Model file for the job. Use its own axes, mm. A direction names the side the tool comes from. Round coordinates to 2 decimals unless told otherwise and drop trailing zeros. Loops run counter-clockwise (first coordinate to the right, second up) from the corner with the lowest first, then second, coordinate; pieces in that order, holes last. Notation, with made-up numbers: M -28,-2 L -17,-2 A21 cw -17,25 Z; hole C 22,58 d5. An arc over 180 degrees is marked long. Use a Markdown table: item, result. Add a question column.
Q1. Cut at A-A (y = 0). Give the cut face in (x, z).
Q2. Mould opens along Y. For faces 6 (the face through (12, 16, 5)), 7 (the face through (5, -7, 29.4)), 8 (the face through (-1, 15, 11.6)) say: +Y half, -Y half, draft (parallel to the pull), parting line (faces both ways), or undercut.
Q3. Pin check, flat tips, straight feed: pin 1 (0.9 mm diameter, centred on x = 6, y = -3, fed in from +Z); pin 2 (5 mm diameter, centred on x = -12.5, z = 8.5, fed in from +Y); pin 3 (8 mm diameter, centred on y = -1, z = 25.5, fed in from +X). Stop position of each tip, or through.
Q4. Probe line 1 (X direction, y = -10, z = 8.75); line 2 (Y direction, x = 0, z = 7); line 3 (Y direction, x = 2, z = 21.75). List the from-to ranges inside material, lowest first. Write a range as from..to.
Q5. Cut at B-B (z = 8.5). Give the cut face in (x, y) (3 decimals).
Q6. Tool access for faces 1 (the face through (-3.5, -6, 28)), 2 (the face through (-1.5, 16.164, 11.5)), 3 (the face through (1.5, 16.164, 11.5)), 4 (the face through (-4.75, 7, 28)), 5 (the face through (6, 0, 9)): list every direction of +Z, -Z, +X, -X, +Y, -Y with a clear straight run to the whole face (end or side of a thin tool).
from build123d import *

# Parameters (mm, degrees)
SKETCH1_R           = 20
SKETCH1_R_2         = 4.75
BOSS_EXTRUDE1_DEPTH = 11
SKETCH2_W           = 13.186598354
SKETCH2_H           = 1
SKETCH2_W_2         = 3
SKETCH2_H_2         = 26.426474467
SKETCH2_H_3         = 26.621798467
SKETCH2_W_3         = 38.736212376
SKETCH2_H_4         = 3
CUT_EXTRUDE1_DEPTH  = 31.347981811
SKETCH3_R           = 2.05
CUT_EXTRUDE2_DEPTH  = 28.766886754
SKETCH5_R           = 0.9
BOSS_EXTRUDE2_DEPTH = 18.4
SKETCH13_R          = 0.9
BOSS_EXTRUDE3_DEPTH = 8.4
SKETCH7_W           = 18.227706113
SKETCH7_H           = 3
CUT_EXTRUDE4_DEPTH  = 1
FILLET1_R           = 7
SKETCH9_R           = 4.5
CUT_EXTRUDE5_DEPTH  = 32.441374016
SKETCH10_R          = 4.75
CUT_EXTRUDE6_DEPTH  = 39.914778684
SKETCH11_W          = 9.5
SKETCH11_H          = 3
CUT_EXTRUDE7_DEPTH  = 7
SKETCH12_R          = 6
CUT_EXTRUDE8_DEPTH  = 14.4
CHAMFER2_SIZE       = 1.5
CHAMFER1_SIZE       = 4
CHAMFER1_SIZE2      = 4.76701437
FILLET2_R           = 10
SKETCH14_W          = 7
SKETCH14_H          = 3
CUT_EXTRUDE9_DEPTH  = 10
BOSS_EXTRUDE4_DEPTH = 1


with BuildPart() as part:
    # Sketch1 → Boss-Extrude1 (new body)
    with BuildSketch(Plane.XY):
        Circle(SKETCH1_R)
        Circle(SKETCH1_R_2, mode=Mode.SUBTRACT)
    extrude(amount=BOSS_EXTRUDE1_DEPTH)

    # Sketch2 → Cut-Extrude1 (cut, through all)
    with BuildSketch(Plane.XY.offset(11)):
        with Locations((0, 19.5)):
            Rectangle(SKETCH2_W, SKETCH2_H)
        with Locations((-18.5, 2.677583481)):
            Rectangle(SKETCH2_W_2, SKETCH2_H_2)
        with Locations((18.5, -1.585343055)):
            Rectangle(SKETCH2_W_2, SKETCH2_H_3)
        with Locations((0.423755219, -18.5)):
            Rectangle(SKETCH2_W_3, SKETCH2_H_4)
    extrude(amount=-CUT_EXTRUDE1_DEPTH, mode=Mode.SUBTRACT)

    # Sketch3 → Cut-Extrude2 (cut, through all)
    with BuildSketch(Plane.XY.offset(11)):
        with Locations((-10.606601718, -10.606601718)):
            Circle(SKETCH3_R)
        with Locations((-10.606601718, 10.606601718)):
            Circle(SKETCH3_R)
        with Locations((10.606601718, 10.606601718)):
            Circle(SKETCH3_R)
        with Locations((10.606601718, -10.606601718)):
            Circle(SKETCH3_R)
    extrude(amount=-CUT_EXTRUDE2_DEPTH, mode=Mode.SUBTRACT)

    # Sketch5 → Boss-Extrude2 (add)
    with BuildSketch(Plane.XY.offset(11)):
        with BuildLine():
            Line((7.5, -5), (7.5, 5))
            ThreePointArc((7.5, 5), (6.328427125, 7.828427125), (3.5, 9))
            Line((3.5, 9), (-3.5, 9))
            ThreePointArc((-3.5, 9), (-6.328427125, 7.828427125), (-7.5, 5))
            Line((-7.5, 5), (-7.5, -5))
            ThreePointArc((-7.5, -5), (-6.328427125, -7.828427125), (-3.5, -9))
            Line((-3.5, -9), (3.5, -9))
            ThreePointArc((3.5, -9), (6.328427125, -7.828427125), (7.5, -5))
        make_face()
        with Locations(Location((-5.75, 0, 0), (0, 0, 180))):
            Circle(SKETCH5_R, mode=Mode.SUBTRACT)
        with Locations(Location((5.75, 0, 0), (0, 0, 180))):
            Circle(SKETCH5_R, mode=Mode.SUBTRACT)
    extrude(amount=BOSS_EXTRUDE2_DEPTH)

    # Sketch13 → Boss-Extrude3 (add)
    with BuildSketch(Plane.XY.offset(11)):
        with Locations(Location((5.75, 0, 0), (0, 0, 180))):
            Circle(SKETCH13_R)
        with Locations(Location((-5.75, 0, 0), (0, 0, 180))):
            Circle(SKETCH13_R)
    extrude(amount=BOSS_EXTRUDE3_DEPTH)

    # Sketch7 → Cut-Extrude4 (cut)
    with BuildSketch(Plane.XY.offset(29.4)):
        with Locations((0.270040091, -3.5)):
            Rectangle(SKETCH7_W, SKETCH7_H)
    extrude(amount=-CUT_EXTRUDE4_DEPTH, mode=Mode.SUBTRACT)

    # Fillet1
    # the kernel refuses this fillet: 7 mm, written as the material it adds along each edge
    with BuildSketch(Plane(origin=(-3.5, -9, 11), x_dir=(0, -1, 0), z_dir=(1, 0, 0)), Plane(origin=(3.5, 9, 11), x_dir=(0, 1, 0), z_dir=(-1, 0, 0))) as fillet1_piece_1:
        with BuildLine():
            CenterArc((FILLET1_R, -FILLET1_R), FILLET1_R, 90, 90)
            Line((0, -FILLET1_R), (0, 0))
            Line((0, 0), (FILLET1_R, 0))
        make_face()
    extrude(amount=7)
    with BuildSketch(Plane(origin=(-3.5, -5, 11), x_dir=(-1, 0, 0), z_dir=(0, 1, 0))) as fillet1_piece_2_section:
        with BuildLine():
            CenterArc((4 + FILLET1_R, FILLET1_R), FILLET1_R, 180, 90)
            Line((4, FILLET1_R), (4, 0))
            Line((4, 0), (4 + FILLET1_R, 0))
        make_face()
    fillet1_piece_2 = revolve(axis=Axis((-3.5, -5, 11), (0, 0, 1)), revolution_arc=90, mode=Mode.PRIVATE)
    fillet1_piece_2 = fillet1_piece_2 - Plane(origin=(-10.606601718, -10.606601718, 12.414511809), x_dir=(1, 0, 0), z_dir=(0, 0, 1)) * Cylinder(2.05, 44, mode=Mode.PRIVATE)
    add(fillet1_piece_2)
    with BuildSketch(Plane(origin=(-7.5, 5, 11), x_dir=(-1, 0, 0), z_dir=(0, -1, 0)), Plane(origin=(7.5, -5, 11), x_dir=(1, 0, 0), z_dir=(0, 1, 0))) as fillet1_piece_3:
        with BuildLine():
            CenterArc((FILLET1_R, -FILLET1_R), FILLET1_R, 90, 90)
            Line((0, -FILLET1_R), (0, 0))
            Line((0, 0), (FILLET1_R, 0))
        make_face()
    extrude(amount=10)
    with BuildSketch(Plane(origin=(-3.5, 5, 11), x_dir=(0, 1, 0), z_dir=(1, 0, 0))) as fillet1_piece_4_section:
        with BuildLine():
            CenterArc((4 + FILLET1_R, FILLET1_R), FILLET1_R, 180, 90)
            Line((4, FILLET1_R), (4, 0))
            Line((4, 0), (4 + FILLET1_R, 0))
        make_face()
    fillet1_piece_4 = revolve(axis=Axis((-3.5, 5, 11), (0, 0, 1)), revolution_arc=90, mode=Mode.PRIVATE)
    fillet1_piece_4 = fillet1_piece_4 - Plane(origin=(-10.606601718, 10.606601718, 12.41451172), x_dir=(1, 0, 0), z_dir=(0, 0, 1)) * Cylinder(2.05, 44, mode=Mode.PRIVATE)
    add(fillet1_piece_4)
    with BuildSketch(Plane(origin=(3.5, 5, 11), x_dir=(1, 0, 0), z_dir=(0, -1, 0))) as fillet1_piece_5_section:
        with BuildLine():
            CenterArc((4 + FILLET1_R, FILLET1_R), FILLET1_R, 180, 90)
            Line((4, FILLET1_R), (4, 0))
            Line((4, 0), (4 + FILLET1_R, 0))
        make_face()
    fillet1_piece_5 = revolve(axis=Axis((3.5, 5, 11), (0, 0, 1)), revolution_arc=90, mode=Mode.PRIVATE)
    fillet1_piece_5 = fillet1_piece_5 - Plane(origin=(10.606601718, 10.606601718, 12.414511728), x_dir=(1, 0, 0), z_dir=(0, 0, 1)) * Cylinder(2.05, 44, mode=Mode.PRIVATE)
    add(fillet1_piece_5)
    with BuildSketch(Plane(origin=(3.5, -5, 11), x_dir=(0, -1, 0), z_dir=(-1, 0, 0))) as fillet1_piece_6_section:
        with BuildLine():
            CenterArc((4 + FILLET1_R, FILLET1_R), FILLET1_R, 180, 90)
            Line((4, FILLET1_R), (4, 0))
            Line((4, 0), (4 + FILLET1_R, 0))
        make_face()
    fillet1_piece_6 = revolve(axis=Axis((3.5, -5, 11), (0, 0, 1)), revolution_arc=90, mode=Mode.PRIVATE)
    fillet1_piece_6 = fillet1_piece_6 - Plane(origin=(10.606601718, -10.606601718, 12.4145119), x_dir=(1, 0, 0), z_dir=(0, 0, 1)) * Cylinder(2.05, 44, mode=Mode.PRIVATE)
    add(fillet1_piece_6)

    # Sketch9 → Cut-Extrude5 (cut, through all)
    with BuildSketch(Plane.XY.offset(11)):
        with Locations((10.606601718, 10.606601718)):
            Circle(SKETCH9_R)
        with Locations((10.606601718, -10.606601718)):
            Circle(SKETCH9_R)
        with Locations((-10.606601718, -10.606601718)):
            Circle(SKETCH9_R)
        with Locations((-10.606601718, 10.606601718)):
            Circle(SKETCH9_R)
    extrude(amount=CUT_EXTRUDE5_DEPTH, mode=Mode.SUBTRACT)

    # Sketch10 → Cut-Extrude6 (cut, through all)
    with BuildSketch(Plane(origin=(0, 0, 0), x_dir=(-1, 0, 0), z_dir=(0, 0, -1))):
        with Locations(Location((0, 0, 0), (0, 0, 335.09893763))):
            Circle(SKETCH10_R)
    extrude(amount=-CUT_EXTRUDE6_DEPTH, mode=Mode.SUBTRACT)

    # Sketch11 → Cut-Extrude7 (cut)
    with BuildSketch(Plane(origin=(0, 9, 0), x_dir=(1, 0, 0), z_dir=(0, 1, 0))):
        with Locations((0, -27.9)):
            Rectangle(SKETCH11_W, SKETCH11_H)
    extrude(amount=-CUT_EXTRUDE7_DEPTH, mode=Mode.SUBTRACT)

    # Sketch12 → Cut-Extrude8 (cut)
    with BuildSketch(Plane(origin=(0, 0, 0), x_dir=(-1, 0, 0), z_dir=(0, 0, -1))):
        Circle(SKETCH12_R)
    extrude(amount=-CUT_EXTRUDE8_DEPTH, mode=Mode.SUBTRACT)

    # Chamfer2
    # the kernel refuses this chamfer: 1.5 mm, written as the material it adds along each edge
    with BuildSketch(Plane(origin=(0, 0, 14.4), x_dir=(-1, 0, 0), z_dir=(0, -1, 0))) as chamfer2_piece_1_section:
        Polygon((6, CHAMFER2_SIZE), (6 - CHAMFER2_SIZE, 0), (6, 0), align=None)
    chamfer2_piece_1 = revolve(axis=Axis((0, 0, 14.4), (0, 0, -1)), mode=Mode.PRIVATE)
    chamfer2_piece_1 = chamfer2_piece_1 - Plane(origin=(0, 0, 13.528251252), x_dir=(-0.9070362073508065, -0.4210526315731381, 0), z_dir=(0, 0, -1)) * Cylinder(4.75, 24, mode=Mode.PRIVATE)
    add(chamfer2_piece_1)

    # Chamfer1
    chamfer1_edges = [part.edges().sort_by_distance(p)[0] for p in [
        (6, 0, 0),
    ]]
    chamfer1_side = [part.faces().sort_by_distance(p)[0] for p in [
        (16.504823264, 0, 0),
    ]]
    chamfer(chamfer1_edges, length=CHAMFER1_SIZE, length2=CHAMFER1_SIZE2, reference=chamfer1_side[0])

    # Fillet2
    # the kernel refuses this fillet: 10 mm, written as the material it adds along each edge
    with BuildSketch(Plane(origin=(4.75, 2, 29.4), x_dir=(-1, 0, 0), z_dir=(0, 0, -1)), Plane(origin=(-4.75, 2, 19.052989911), x_dir=(1, 0, 0), z_dir=(0, 0, 1))) as fillet2_piece_1:
        with BuildLine():
            CenterArc((10, 2.938804035), FILLET2_R, 180, 17.090413612)
            Line((0, 2.938804035), (-0.2, 2.938804035))
            Line((-0.2, 2.938804035), (-0.2, 0))
            Line((-0.2, 0), (0, -0.2))
            ThreePointArc((0, -0.2), (0.220789008, -0.2), (0.250409575, -0.058776081))
            Line((0.250409575, -0.058776081), (0.441578015, 0))
        make_face()
    extrude(amount=10.347010089)

    # Sketch14 → Cut-Extrude9 (cut)
    with BuildSketch(Plane.XZ.offset(9)):
        with Locations((0, 27.9)):
            Rectangle(SKETCH14_W, SKETCH14_H)
    extrude(amount=-CUT_EXTRUDE9_DEPTH, mode=Mode.SUBTRACT)

    # Sketch15 → Boss-Extrude4 (add)
    with BuildSketch(Plane.XY.offset(11)):
        Polygon((-1, 13.002035862), (1, 13.002035862), (1, 16.164200489), (2, 16.164200489), (0, 18.664200489), (-2, 16.164200489), (-1, 16.164200489), align=None)
    extrude(amount=BOSS_EXTRUDE4_DEPTH)


solid = part.part
Checked values:
| question | item | result |
|---|---|---|
| 1 | outline | M -17,0 L -10,0 L -6,4.77 L -6,12.9 L -4.75,14.15 L -4.75,29.4 L -4.85,29.4 L -4.85,19.4 L -6.65,19.4 L -6.65,29.4 L -7.5,29.4 L -7.5,18 A7 cw -14.5,11 L -17,11 Z; M 4.75,14.15 L 6,12.9 L 6,4.77 L 10,0 L 17,0 L 17,11 L 14.5,11 A7 cw 7.5,18 L 7.5,29.4 L 6.65,29.4 L 6.65,19.4 L 4.85,19.4 L 4.85,29.4 L 4.75,29.4 Z |
| 2 | face 6 | +Y half |
| 2 | face 7 | draft |
| 2 | face 8 | undercut |
| 3 | pin 1 | stops at z = 28.4 |
| 3 | pin 2 | stops at y = 17.32 |
| 3 | pin 3 | stops at x = 7.5 |
| 4 | line 1 | x = -17..-12.56, -8.65..8.65, 12.56..17 |
| 4 | line 2 | y = -17..-6, 6..19 |
| 4 | line 3 | y = -9..-4.31, 4.31..9 |
| 5 | outline | M -17,-10.536 A20 ccw -10.536,-17 L 10.536,-17 A20 ccw 17,-10.536 L 17,10.536 A20 ccw 6.245,19 L -6.245,19 A20 ccw -17,10.536 Z; hole C -10.607,-10.607 d4.1; hole C -10.607,10.607 d4.1; hole C 0,0 d12; hole C 10.607,-10.607 d4.1; hole C 10.607,10.607 d4.1 |
| 6 | face 1 | +Z, +Y, -Y |
| 6 | face 2 | +Z, -X |
| 6 | face 3 | +Z, +X |
| 6 | face 4 | +Z, +Y |
| 6 | face 5 | -Z |
